Input: part model. Units: mm. Frame: model coordinates. Coordinates: 2 decimals unless noted, no trailing zeros. Order: outer loops, then holes, each group sorted by start corner. A loop starts at its lowest first (then second) coordinate and runs counter-clockwise, first axis right, second up.
from build123d import *

# Parameters (mm, degrees)
F1_DEPTH = 1.6
F2_D     = 8


with BuildPart() as f1:
    # F0 (on Front) → F1 (new body)
    with BuildSketch(Plane.XZ):
        Polygon((180, 0), (0, 0), (0, -300), (270, -300), (270, -250), (180, -250), align=None)
    extrude(amount=F1_DEPTH)

    # F2 (through all)
    with Locations(Plane(origin=(0, 0, 0), x_dir=(1, 0, 0), z_dir=(0, 1, 0))):
        with Locations((15, 75), (48, 285), (168, 285)):
            Hole(F2_D / 2)


solid = f1.part
Item 1: Cut plane C-C on z = -230. Return loops of the section in (x, y), then the cut area to 3 significant figures.
Response values:
outline: (0, -1.6) - (180, -1.6) - (180, 0) - (0, 0) - close
area: 288 mm2
Item 2: Ray query, probe 1 along X at (y, z) = (-0.8, -285); probe 2 along Z at (x, y) = (15, -0.8); probe 3 along Z at (x, y) = (48, -0.5). Return the intervals inside material, ascending.
Response values:
probe 1: x = 0 to 44, 52 to 164, 172 to 270
probe 2: z = -300 to -79, -71 to 0
probe 3: z = -300 to -289, -281 to 0
Item 3: Draft query along X for faces 1 (the face through (103, -1.6, -148)), 2 (the face through (166.154, -0.811, -281.451)). Return one class per face: pulls with the +X half, pulls with the -X half, needs draft (parallel to the pull), parting line crosses it, or undercut.
Response values:
face 1: needs draft
face 2: undercut
Item 4: Cut plane A-A on x = 48. Return loops of the section in (y, z), then the cut area to 3 significant figures.
Response values:
outline: (-1.6, -300) - (0, -300) - (0, -289) - (-1.6, -289) - close; (-1.6, -281) - (0, -281) - (0, 0) - (-1.6, 0) - close
area: 467 mm2
Item 5: Pin query (flat end, axial travel): pin 1 Ø0.5 at (x, y) = (244, -1) entering from +Z. Return the tip coordinate at first contact, or that it passes through.
Response values:
pin 1: stops at z = -250
Item 6: Cut plane D-D on x = 226.5. Return loops of the section in (y, z), then the cut area to 3 significant figures.
Response values:
outline: (-1.6, -300) - (0, -300) - (0, -250) - (-1.6, -250) - close
area: 80.0 mm2
Item 7: Cut plane B-B on y = -1.2. Return loops of the section in (x, z), then the cut area to 3 significant figures.
Response values:
outline: (0, -300) - (270, -300) - (270, -250) - (180, -250) - (180, 0) - (0, 0) - close; hole circle Ø8 at (15, -75); hole circle Ø8 at (48, -285); hole circle Ø8 at (168, -285)
area: 58,300 mm2
